Autodesk Fusion 360 part; units mm, degrees
sketch "Skizze1" plane through (0, 0, 0) normal (0, 0, 1) x (1, 0, 0)
  circle A0 centre (0, 0) radius 130
  dimension "d1" = 260
extrude "Extrusion1" add sketch "Skizze1" along normal blind 3
sketch "Skizze3" plane through (0, 0, 0) normal (0, 0, -1) x (1, 0, 0)
  circle A0 centre (0, 0) radius 130
  circle A1 centre (-85, 85) radius 1.5
  circle A2 centre (-85, -85) radius 1.5
  circle A3 centre (85, -85) radius 1.5
  circle A4 centre (85, 85) radius 1.5
  dimension "d4" = 3
  dimension "d5" = 85
  dimension "d6" = 85
  dimension "d8" = 360
extrude "Extrusion2" cut sketch "Skizze3" against normal blind 3 contours A1 | A2 | A3 | A4
chamfer "Fase1" distance 1.5 angle 45 4 edges at (-86.3985, -85.5424, 0) (83.6015, -85.5424, 0) (-86.3985, 84.4576, 0) (83.6015, 84.4576, 0)
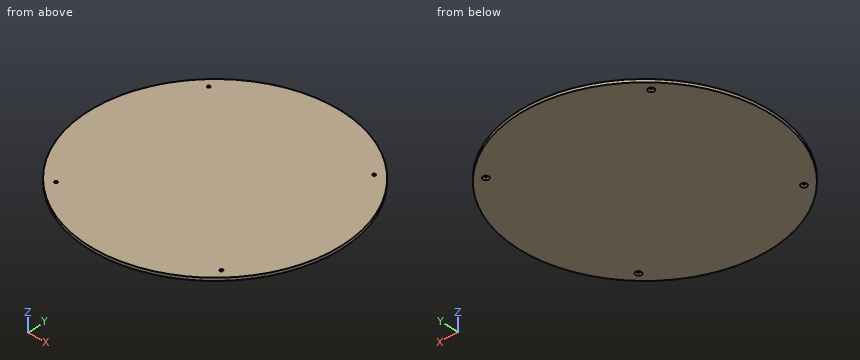
Model file for the job. Use its own axes, mm. Coordinates: 2 decimals unless noted, no trailing zeros. Order: outer loops, then holes, each group sorted by start corner. A loop starts at its lowest first (then second) coordinate and runs counter-clockwise, first axis right, second up. Notation, with made-up numbers: (34, -28.5) -> (45, -28.5) arc R13 cw to (45, -8.5) -> close; hole circle Ø7 at (-9.5, -23). An arc over 180 degrees is marked (long way). Return JSON: item names as keys, results as strings. Group by question number.
Item 1: Saw through at B-B on x = -36.5. Write the cut outline in (y, z).
Item 2: Saw through at C-C on y = -41.5. Write the cut outline in (x, z).
Item 3: Wall check: line 1 along X through (y, z) = (-85, 2.65); line 2 along X through (y, z) = (-104, 0.4). Give the ranges that are in metal, low to high. Write a range as [from, to].
Item 4: Flat gauge pins, fed straight in: P1, Ø1.5, axis at x = -31, z = 2.5, coming from the -Y side; P2, Ø3.5, axis at x = 85, y = -85, coming from the -Z side. Where does each tip first touch, or does it go through?
Item 5: Saw through at A-A on z = 0.85. Write the cut outline in (x, y), then the cut area to 3 significant figures.
Values found:
{
 "1": {"outline": "(-124.77, 0) -> (124.77, 0) -> (124.77, 3) -> (-124.77, 3) -> close"},
 "2": {"outline": "(-123.2, 0) -> (123.2, 0) -> (123.2, 3) -> (-123.2, 3) -> close"},
 "3": {"line 1": "x = [-98.36, -86.5], [-83.5, 83.5], [86.5, 98.36]", "line 2": "x = [-78, 78]"},
 "4": {"P1": "stops at y = -126.43", "P2": "stops at z = 1.25"},
 "5": {"outline": "circle Ø260 at (0, 0); hole circle Ø4.3 at (-85, -85); hole circle Ø4.3 at (-85, 85); hole circle Ø4.3 at (85, -85); hole circle Ø4.3 at (85, 85)", "area": "53,000 mm2"}
}
